Input: part model. Units: mm. Frame: model coordinates. A direction names the side the tool comes from. Give positions to 0.01 mm unless a question says otherwise; leave off trailing zeros. Loops run counter-clockwise (first coordinate to the right, second up) from the corner with the lowest first, then second, coordinate; pieces in that order, holes last. Notation, with made-up numbers: (0.25, 7) -> (16.25, 7) arc R15 ccw to (16.25, 31) -> close; hole circle Ø2 at (12, 11). An arc over 180 degrees is marked (long way). Answer as a JSON object with one key per item and string values.
```python
from build123d import *

# Parameters (mm, degrees)
SKETCH_1_R               = 5
EXTRUDE_1_DEPTH          = 4
SKETCH_4_R               = 2.5
EXTRUDE_2_DEPTH          = 4
SKETCH_2_R               = 1.5
CUT_EXTRUDE_1_DEPTH      = 4
CUT_EXTRUDE_1_DEPTH_BACK = 3
SKETCH_3_R               = 4.05
CUT_EXTRUDE_2_DEPTH      = 3


with BuildPart() as part:
    # 草图1 → 凸台-拉伸1 (new body)
    with BuildSketch(Plane.XY):
        Circle(SKETCH_1_R)
    extrude(amount=EXTRUDE_1_DEPTH)

    # 草图4 → 凸台-拉伸2 (add)
    with BuildSketch(Plane(origin=(0, 0, 0), x_dir=(-1, 0, 0), z_dir=(0, 0, -1))):
        Circle(SKETCH_4_R)
    extrude(amount=EXTRUDE_2_DEPTH)

    # 草图2 → 切除-拉伸1 (cut, two sides)
    with BuildSketch(Plane(origin=(0, 0, 0), x_dir=(-1, 0, 0), z_dir=(0, 0, -1))) as cut_extrude_1_sk:
        Circle(SKETCH_2_R)
    extrude(amount=CUT_EXTRUDE_1_DEPTH, mode=Mode.SUBTRACT)
    extrude(cut_extrude_1_sk.sketch, amount=-CUT_EXTRUDE_1_DEPTH_BACK, mode=Mode.SUBTRACT)

    # 草图3 → 切除-拉伸2 (cut)
    with BuildSketch(Plane.XY.offset(4)):
        Circle(SKETCH_3_R)
    extrude(amount=-CUT_EXTRUDE_2_DEPTH, mode=Mode.SUBTRACT)


solid = part.part
```
Q1. Section A-A, the plane y = 0. Return the cut outline in (x, z), then the cut area to 3 significant figures.
Evaluation:
{"outline": "(-5, 0) -> (-2.5, 0) -> (-2.5, -4) -> (-1.5, -4) -> (-1.5, 1) -> (-4.05, 1) -> (-4.05, 4) -> (-5, 4) -> close; (1.5, -4) -> (2.5, -4) -> (2.5, 0) -> (5, 0) -> (5, 4) -> (4.05, 4) -> (4.05, 1) -> (1.5, 1) -> close", "area": "20.7 mm2"}
Q2. Ray query, line 1 along Y through (x, z) = (0, 2.1); line 2 along Y through (x, z) = (0, -2.8); line 3 along Y through (x, z) = (-2, -0.75). Return the intervals inside material, ascending.
Evaluation:
{"line 1": "y = -5 to -4.05, 4.05 to 5", "line 2": "y = -2.5 to -1.5, 1.5 to 2.5", "line 3": "y = -1.5 to 1.5"}
Q3. Access query for faces 4 (the cylindrical face through (-0.878, -3.954, 2.521)), 5 (the cylindrical face through (1.5, 0.07, -1.46)), 6 (the flat face through (2, -2, 0)). Directions: +Z, -Z, +X, -X, +Y, -Y. A direction counts if a zero-diameter tool reaches every point of the face in a straight line with its end or side. Return the directions, or none.
Evaluation:
{"face 4": "+Z", "face 5": "+Z, -Z", "face 6": "-Z"}
Q4. Section C-C, the plane z = 0.5. Return the cut outline in (x, y).
Evaluation:
{"outline": "circle Ø10 at (0, 0); hole circle Ø3 at (0, 0)"}
Q5. Pin query (flat end, axial travel): pin 1 (1 mm diameter, centred on x = 1, y = -1.5, fed in from +Z); pin 2 (2 mm diameter, centred on x = 2, z = 2, fed in from +Y); pin 3 (2.5 mm diameter, centred on x = 0, y = 0, fed in from +Z); pin 4 (1.5 mm diameter, centred on y = -2, z = -1, fed in from -X). Return the tip coordinate at first contact, or that it passes through.
Evaluation:
{"pin 1": "stops at z = 1", "pin 2": "stops at y = 4.9", "pin 3": "passes through", "pin 4": "stops at x = -2.17"}
Q6. Draft query along Y for faces 1 (the cylindrical face through (0.54, -2.44, -1.97)), 2 (the flat face through (0, -2, -4)), 3 (the flat face through (2, 0, 1)). Return one class per face: +Y half, -Y half, draft (parallel to the pull), parting line (faces both ways), or undercut.
Evaluation:
{"face 1": "parting line", "face 2": "draft", "face 3": "undercut"}
Q7. Section D-D, the plane y = 3.5. Return the cut outline in (x, z).
Evaluation:
{"outline": "(-3.57, 0) -> (3.57, 0) -> (3.57, 4) -> (2.04, 4) -> (2.04, 1) -> (-2.04, 1) -> (-2.04, 4) -> (-3.57, 4) -> close"}
